Autodesk Inventor part; units mm, degrees
ref_plane "YZ Plane" through (0, 0, 0) normal (1, 0, 0) x (0, 1, 0)
ref_plane "XZ Plane" through (0, 0, 0) normal (0, 1, 0) x (-1, 0, 0)
ref_plane "XY Plane" through (0, 0, 0) normal (0, 0, 1) x (1, 0, 0)
sketch "Boceto1" plane through (0, 0, 0) normal (0, 1, 0) x (-1, 0, 0)
  line L0 (0, 0) -> (12.5, 0)
  line L1 (12.5, 0) -> (12.5, 5)
  line L2 (12.5, 5) -> (0, 5)
  line L3 (0, 5) -> (0, 0)
  circle A0 centre (6.25, 2.5) radius 1
  arc A1 (8.4861, 0) -> (4.0139, 0) centre (6.25, -2) ccw
  circle A2 centre (6.25, -25) radius 1
  line L4 (6.25, -25) -> (6.25, -22.5)
  line L5 (0, -22.5) -> (12.5, -22.5)
  line L6 (12.5, -22.5) -> (12.5, -27.5)
  line L7 (12.5, -27.5) -> (0, -27.5)
  line L8 (0, -27.5) -> (0, -22.5)
  line L9 (6.25, 0) -> (6.25, -6.25)
  arc A3 (12.5, -6.25) -> (0, -6.25) centre (6.25, -6.25) ccw
  arc A4 (0, -10.25) -> (12.5, -10.25) centre (6.25, -10.25) ccw
  line L10 (12.5, -10.25) -> (12.5, -6.25)
  line L11 (0, -10.25) -> (0, -6.25)
  circle A5 centre (6.25, -6.25) radius 27
  circle A6 centre (6.25, -6.25) radius 30
  dimension "d0" = 12.5
  dimension "d1" = 5
  dimension "d2" = 2
  dimension "d4" = 6
  dimension "d6" = 2
  dimension "d7" = 2.5
  dimension "d8" = 12.5
  dimension "d9" = 5
  dimension "d10" = 6.25
  dimension "d11" = 12.5
  dimension "d13" = 12.5
  dimension "d14" = 54
  dimension "d15" = 60
extrude "Extrusión1" add sketch "Boceto1" along normal blind 3 contours A5
extrude "Extrusión2" add sketch "Boceto1" along normal blind 6.8 contours A6
extrude "Extrusión3" add sketch "Boceto1" against normal blind 5 contours L3 L2 L1 L0 A1 | L5 L6 L7 L8
sketch "Boceto2" plane through (0, 0, 0) normal (0, 1, 0) x (1, 0, 0)
  line L0 (-4.0139, 0) -> (0, 0)
  arc A0 (-8.4861, 0) -> (-4.0139, 0) centre (-6.25, 2) ccw
  line L1 (-12.5, 0) -> (-8.4861, 0)
  line L2 (-12.5, -5) -> (-12.5, 0)
  line L3 (0, -5) -> (-12.5, -5)
  line L4 (0, 0) -> (0, -5)
  circle A1 centre (-6.25, -2.5) radius 1
  line L5 (0, 27.5) -> (0, 22.5)
  line L6 (-12.5, 27.5) -> (0, 27.5)
  line L7 (-12.5, 22.5) -> (-12.5, 27.5)
  line L8 (0, 22.5) -> (-12.5, 22.5)
  circle A2 centre (-6.25, 25) radius 1
  line L9 (-12.5, -5) -> (-12.5, 0)
  line L10 (-6.25, 0) -> (0, 0)
  line L11 (-12.5, -5) -> (0, -5)
  line L12 (0, -5) -> (0, 0)
  line L13 (-12.5, 0) -> (-12.5, -5)
  line L14 (-12.5, 27.5) -> (0, 27.5)
  line L15 (0, 22.5) -> (-12.5, 22.5)
  line L16 (0, 27.5) -> (-12.5, 27.5)
  line L17 (-12.5, 27.5) -> (-12.5, 22.5)
  line L18 (-12.5, 22.5) -> (0, 22.5)
  line L19 (0, 22.5) -> (0, 27.5)
  circle A3 centre (-6.25, -2.5) radius 1
  circle A4 centre (-6.25, 25) radius 1
  arc A5 (-8.4861, 0) -> (-4.0139, 0) centre (-6.25, 2) ccw
  line L20 (0, 0) -> (-4.0139, 0)
  line L21 (-8.4861, 0) -> (-12.5, 0)
  line L22 (-8.4861, 0) -> (-4.0139, 0)
  point P0 (-8.4861, 0)
  dimension "d22" = 2
  dimension "d23" = 2
  dimension "d24" = 6
extrude "Extrusión4" add sketch "Boceto2" along normal blind 3
sketch "Boceto3" plane through (-6.25, 0, -6.25) normal (0, -1, 0) x (1, 0, 0)
  circle A0 centre (0, 0) radius 30
  circle A1 centre (0, 0) radius 27
  point P0 (6.25, 6.25)
  dimension "d27" = 60
  dimension "d28" = 54
extrude "Extrusión5" add sketch "Boceto3" along normal blind 25
sketch "Boceto4" plane through (-6.25, -25, -6.25) normal (0, -1, 0) x (1, 0, 0)
  circle A0 centre (0, 0) radius 30
  circle A1 centre (0, 0) radius 27
  circle A2 centre (0, 40) radius 2.5
  arc A3 (3.3493, 42.1868) -> (-3.3436, 42.1955) centre (0, 40) ccw
  circle A4 centre (40, 0) radius 2.5
  arc A5 (42.2251, -3.324) -> (42.295, 3.2761) centre (40, 0) ccw
  circle A6 centre (0, -40) radius 2.5
  arc A7 (-3.111, -42.5143) -> (3.3503, -42.1853) centre (0, -40) ccw
  circle A8 centre (-40, 0) radius 2.5
  arc A9 (-42.5143, 3.111) -> (-42.5143, -3.111) centre (-40, 0) ccw
  line L0 (-3.995, 39.8) -> (-3.995, 39.8)
  arc A10 (3.3493, 42.1868) -> (5.8327, 39.5725) centre (11.7225, 47.6539) ccw
  arc A11 (-5.8604, 39.5684) -> (-3.3436, 42.1955) centre (-11.7026, 47.6843) ccw
  arc A12 (39.5114, 6.2326) -> (5.8327, 39.5725) centre (0, 0) ccw
  arc A13 (5.8279, -39.5732) -> (39.5535, -5.9597) centre (0, 0) ccw
  arc A14 (-5.8604, 39.5684) -> (-39.04, 8.7108) centre (0, 0) ccw
  arc A15 (-39.04, -8.7108) -> (-8.7108, -39.04) centre (0, 0) ccw
  line L1 (-3.995, -39.8) -> (-6.9108, -38.8236)
  line L2 (8.3455, -38.2373) -> (8.1717, -38.2997)
  arc A16 (42.2251, -3.324) -> (39.5535, -5.9597) centre (47.7877, -11.6341) ccw
  arc A17 (39.5114, 6.2326) -> (42.295, 3.2761) centre (48.0324, 11.4665) ccw
  arc A18 (5.8279, -39.5732) -> (3.3503, -42.1853) centre (11.726, -47.6486) ccw
  arc A19 (-3.111, -42.5143) -> (-8.7108, -39.04) centre (-10.8885, -48.8) ccw
  arc A20 (-42.5143, 3.111) -> (-39.04, 8.7108) centre (-48.8, 10.8885) ccw
  arc A21 (-39.04, -8.7108) -> (-42.5143, -3.111) centre (-48.8, -10.8885) ccw
  point P0 (6.25, 6.25)
  dimension "d32" = 60
  dimension "d33" = 54
  dimension "d34" = 5
  dimension "d35" = 8
  dimension "d36" = 5
  dimension "d37" = 8
  dimension "d38" = 5
  dimension "d39" = 8
  dimension "d40" = 5
  dimension "d41" = 8
  dimension "d42" = 10
  dimension "d43" = 10
extrude "Extrusión6" add sketch "Boceto4" along normal blind 3 contours A0 | A10 A12 A17 A5 A16 A13 A18 A7 A19 A15 A21 A9 A20 A14 A11 A3
sketch "Boceto5" plane through (0, 0, 0) normal (0, 0, 1) x (1, 0, 0)
  line L0 (-2.9007, -25) -> (-9.5936, -25)
  line L1 (-9.5936, -25) -> (-9.5936, -28)
  line L2 (-2.9007, -28) -> (-9.5936, -28)
  line L3 (-2.9007, -25) -> (-2.9007, -28)
  line L4 (-9.5936, -25) -> (-12.1104, -25)
  line L5 (-12.1104, -25) -> (-12.1104, -28)
  line L6 (-9.5936, -28) -> (-12.1104, -28)
  line L7 (-9.5936, -25) -> (-9.5936, -28)
  line L8 (-0.4173, -25) -> (-2.9007, -25)
  line L9 (-2.9007, -25) -> (-2.9007, -28)
  line L10 (-0.4173, -28) -> (-2.9007, -28)
  line L11 (-0.4173, -25) -> (-0.4173, -28)
  line L12 (-6.2472, -25) -> (-1.2472, -25)
  line L13 (-0.4173, -25) -> (-2.9007, -25)
  line L14 (-1.2472, -25) -> (-11.2472, -25)
  line L15 (-11.2472, -25) -> (-1.2472, -25)
  line L16 (-1.2472, -25) -> (-1.2472, -20)
  line L17 (-1.2472, -20) -> (-11.2472, -20)
  line L18 (-11.2472, -20) -> (-11.2472, -25)
  point P0 (0, 0)
  dimension "d46" = 5
  dimension "d47" = 10
  dimension "d48" = 10
  dimension "d49" = 5
extrude "Extrusión7" cut sketch "Boceto5" along normal blind 40 contours L0 L4 L18 L17 L16 L8
properties part number "sombreronuevasversionsanti"
Check sheet for the modelled part. Datum: model origin and axes. Units: mm. A direction names the side the tool comes from. Coordinates: 2 decimals unless noted, no trailing zeros. Order: outer loops, then holes, each group sorted by start corner. A loop starts at its lowest first (then second) coordinate and runs counter-clockwise, first axis right, second up. Notation, with made-up numbers: M 73,34 L 97,34 A21 ccw 97,38 Z; hole C 37.25,5.5 d2. An arc over 180 degrees is marked long. Write each question's results on one line, items separated by ' | '. Start each with the question number.
1. Material ranges on probe 1 along Z at (x, y) = (-6.25, -3.95); probe 2 along Z at (x, y) = (-6.25, -25.65); probe 3 along Y at (x, z) = (7.5, 7.5), recorded low to high.
2. Mould release check, pull along Z, two halves, no side actions. Record for faces 1 (the face through (-10, -2, 0)), 2 (the face through (37.75, -26.48, -6.24)), 3 (the face through (-6.3, -26.48, 37.75)), 4 (the face through (-1.8, -26.48, -47.04)): +Z half, -Z half, draft (parallel to the pull), parting line (faces both ways), or undercut.
3. Cross-section at C-C on z = 14. Record the cut outline in (x, y).
4. Cross-section at A-A on y = -15. Record the cut outline in (x, z).
5. Cross-section at D-D on x = -40. Record the cut outline in (y, z), and give its area (3 significant figures).
6. Cross-section at B-B on x = -24.5. Record the cut outline in (y, z).
7. Go/stop test with flat-tipped pins: P1, Ø2.5, axis at x = -6.25, z = -25, coming from the -Y side; P2, Ø10, axis at x = -2, y = -14.5, coming from the -Z side; P3, Ø10, axis at x = -25.5, z = 21.5, coming from the +Y side; P4, Ø3, axis at y = -22.5, z = -29, coming from the -X side. Record where each tip stops, or that it passes through.
8. Access from +Z, -Z, +X, -X, +Y, -Y to the whole of each face (thin tool, end or side, straight path). Record for faces 5 (the face through (-2, -2, 0)), 6 (the face through (-6, -20, 22)), 7 (the face through (0, 1, -8)).
Checks:
1) probe 1: z = -36.25 to -33.25, -27.5 to -26, -24 to -22.5, 1 to 1.5, 3.5 to 5, 20.75 to 23.75 | probe 2: z = -50.25 to -48.75, -43.75 to -33.25, 20.75 to 31.25, 36.25 to 37.75 | probe 3: y = 0 to 3
2) face 1: undercut | face 2: parting line | face 3: +Z half | face 4: -Z half
3) outline: M -40.75,-28 L -24.11,-28 L -24.11,0 L 11.61,0 L 11.61,-28 L 28.25,-28 L 28.25,-25 L 15.88,-25 L 15.88,6.8 L 11.61,6.8 L 11.61,3 L -24.11,3 L -24.11,6.8 L -28.38,6.8 L -28.38,-25 L -40.75,-25 Z
4) outline: C -6.25,-6.25 d60; hole C -6.25,-6.25 d54
5) outline: M -28,-27.72 L -25,-27.72 L -25,15.22 L -28,15.22 Z | area: 129 mm²
6) outline: M -28,-41.84 L -25,-41.84 L -25,-30.06 L 6.8,-30.06 L 6.8,-26.15 L 3,-26.15 L 3,13.65 L 6.8,13.65 L 6.8,17.56 L -25,17.56 L -25,29.34 L -28,29.34 L -28,13.65 L 0,13.65 L 0,-26.15 L -28,-26.15 Z
7) P1: stops at y = -5 | P2: stops at z = -36.25 | P3: stops at y = 6.8 | P4: stops at x = -27.43
8) face 5: -Y | face 6: +Z | face 7: +Y, -Y
